```python
from build123d import *

# Parameters (mm, degrees)
SKETCH002_W     = 15
SKETCH002_H     = 6
PAD_DEPTH       = 2
PAD_DEPTH_BACK  = 5
POCKET_DEPTH    = 5.001
POCKET001_DEPTH = 2.001


with BuildPart() as part:
    # Sketch002 → Pad (new body, two sides)
    with BuildSketch(Plane.XZ) as pad_sk:
        Rectangle(SKETCH002_W, SKETCH002_H)
    extrude(amount=PAD_DEPTH)
    extrude(pad_sk.sketch, amount=-PAD_DEPTH_BACK)

    # Sketch → Pocket (cut, through all)
    with BuildSketch(Plane.XZ):
        with BuildLine():
            ThreePointArc((-2.95, 1.65), (-4.6, 0), (-2.95, -1.65))
            Line((-2.95, -1.65), (2.95, -1.65))
            ThreePointArc((2.95, -1.65), (4.6, 0), (2.95, 1.65))
            Line((-2.95, 1.65), (2.95, 1.65))
        make_face()
    extrude(amount=-POCKET_DEPTH, mode=Mode.SUBTRACT)

    # Sketch001 → Pocket001 (cut, through all)
    with BuildSketch(Plane.XZ):
        with BuildLine():
            ThreePointArc((-2.85, 1.35), (-4.2, 0), (-2.85, -1.35))
            Line((-2.85, -1.35), (2.85, -1.35))
            ThreePointArc((2.85, -1.35), (4.2, 0), (2.85, 1.35))
            Line((-2.85, 1.35), (2.85, 1.35))
        make_face()
    extrude(amount=POCKET001_DEPTH, mode=Mode.SUBTRACT)


solid = part.part
```
Here's how the part is built. I have some questions about the finished solid (model axes, mm). A direction names the side the tool comes from. Coordinates: 2 decimals unless noted, no trailing zeros. Order: outer loops, then holes, each group sorted by start corner. A loop starts at its lowest first (then second) coordinate and runs counter-clockwise, first axis right, second up.
1) Imagine slicing it at B-B on x = 1.75. List the corners of the cut face in (y, z) for me.
2) Imagine slicing it at C-C on y = 0.5. List the corners of the cut face in (x, z) for me, and give its area (3 significant figures).
3) We'd pull the mould along X, two halves only. Please class faces 4 (the face through (4.2, -1, 0)), 5 (the face through (0, 1, 3)), 6 (the face through (-7.5, 1, 0)), 7 (the face through (0, 2, 1.65)): +X half, -X half, draft (parallel to the pull), parting line (faces both ways), or undercut.
4) Imagine slicing it at A-A on z = 0. List the corners of the cut face in (x, y) for me.
5) I need wall thicknesses on line 1 (Z direction, x = 1.25, y = 0.25); line 2 (Z direction, x = -0.25, y = -1.5); line 3 (X direction, y = 4.5, z = 0.8). Which ranges of each line are inside material? Lowest first, please.
6) Which directions (+Z, -Z, +X, -X, +Y, -Y) give clear straight access to the entire face, cutting with the end or side of a thin tool? Please do faces 1 (the face through (-4.2, -1, 0)), 2 (the face through (0, -2, 2)), 3 (the face through (4.6, 2.5, 0)).
7) Will these pins go through, and if not, where does the flat tip stop? pin 1 (1.5 mm diameter, centred on x = -3.5, z = -1.5, fed in from +Y); pin 2 (1.5 mm diameter, centred on x = 1.5, z = 0, fed in from -Y).
Response values:
1. outline: (-2, -3) - (5, -3) - (5, -1.65) - (0, -1.65) - (0, -1.35) - (-2, -1.35) - close; (-2, 1.35) - (0, 1.35) - (0, 1.65) - (5, 1.65) - (5, 3) - (-2, 3) - close
2. outline: (-7.5, -3) - (7.5, -3) - (7.5, 3) - (-7.5, 3) - close; hole (-2.95, -1.65) - (2.95, -1.65) arc R1.65 ccw to (2.95, 1.65) - (-2.95, 1.65) arc R1.65 ccw to start
2. area: 62.0 mm2
3. face 4: undercut
3. face 5: draft
3. face 6: -X half
3. face 7: undercut
4. outline: (-7.5, -2) - (-4.2, -2) - (-4.2, 0) - (-4.6, 0) - (-4.6, 5) - (-7.5, 5) - close; (4.2, -2) - (7.5, -2) - (7.5, 5) - (4.6, 5) - (4.6, 0) - (4.2, 0) - close
5. line 1: z = -3 to -1.65, 1.65 to 3
5. line 2: z = -3 to -1.35, 1.35 to 3
5. line 3: x = -7.5 to -4.39, 4.39 to 7.5
6. face 1: +Y, -Y
6. face 2: +Z, -Z, +X, -X, -Y
6. face 3: +Y
7. pin 1: stops at y = 5
7. pin 2: passes through
